Can you work these out from the model? Positions are in its coordinate system, mm. A direction names the side the tool comes from. Round coordinates to 2 decimals unless told otherwise and drop trailing zeros. Loops run counter-clockwise (first coordinate to the right, second up) from the corner with the lowest first, then second, coordinate; pieces in that order, holes last. Notation, with made-up numbers: M -39,-19.5 L -24,-19.5 A21 cw -24,14.5 Z; hole C 14,24.25 d10. An arc over 180 degrees is marked long. Return JSON: item names as keys, results as strings.
```python
from build123d import *

# Parameters (mm, degrees)
CYLINDER003_R           = 1.5
CYLINDER003_DEPTH       = 22
BODY002_PLACEMENT_ANGLE = 180
CYLINDER002_R           = 2
CYLINDER002_DEPTH       = 3


with BuildPart() as cylinder003:
    # Cylinder003 → Cylinder003 (new body)
    with BuildSketch(Plane(origin=(18, 0, 0), x_dir=(0, 0, -1), z_dir=(1, 0, 0))):
        Circle(CYLINDER003_R)
    extrude(amount=CYLINDER003_DEPTH)


with BuildPart() as body002:
    # Sketch002 → Revolution002 (revolve)
    with BuildSketch(Plane.XY):
        Polygon((0, 1.5), (0, 13), (-2, 15), (-8, 15), (-8, 14), (-9, 14), (-9, 12), (-5, 12), (-5, 1.5), align=None)
    revolve(axis=Axis((0, 0, 0), (1, 0, 0)))


with BuildPart() as body002_1:
    # Body002 placement: moved
    add(body002.part.moved(Location((12, 0, 0))).rotate(Axis((12, 0, 0), (0, 0, 1)), BODY002_PLACEMENT_ANGLE))


with BuildPart() as cut:
    # Cylinder002 → Cylinder002 (new body)
    with BuildSketch(Plane(origin=(9, 0, 0), x_dir=(0, 0, -1), z_dir=(1, 0, 0))):
        Circle(CYLINDER002_R)
    extrude(amount=CYLINDER002_DEPTH)

    # Fusion: union Body002
    add(body002_1.part)


with BuildPart() as cut_1:
    # Fusion placement: moved
    add(cut.part.moved(Location((11, 0, 0))))

    # Cut: cut Cylinder003
    add(cylinder003.part, mode=Mode.SUBTRACT)


solid = cut_1.part
```
Q1. Suppose I cut it at B-B, the plane x = 26.25. Please give me the cut outline in (y, z).
Results:
{"outline": "C 0,0 d30; hole C 0,0 d3"}
Q2. I'm going to push flat-ended pins straight in: pin 1 Ø3.5 at (y, z) = (0, 0) entering from +X; pin 2 Ø2 at (x, y) = (28, -5.5) entering from -Z; pin 3 Ø1.5 at (x, z) = (27, 1.5) entering from +Y; pin 4 Ø8 at (y, z) = (9, -4) entering from +X. Where does each tip first touch, or does it pass through?
Results:
{"pin 1": "stops at x = 28", "pin 2": "stops at z = -14.31", "pin 3": "stops at y = 14.98", "pin 4": "stops at x = 32"}
Q3. If I drill on line 1 along Y through (x, z) = (21.4, 0); line 2 along Z through (x, y) = (29.8, 0); line 3 along X through (y, z) = (9, 6), over which ranges is the centre line in solid material (lowest first)?
Results:
{"line 1": "y = -2 to -1.5, 1.5 to 2", "line 2": "z = -15 to -12, 12 to 15", "line 3": "x = 23 to 28"}
Q4. On a 3-axis mill with a long thin cutter (end or side, diameter ignored), from which of +Z, -Z, +X, -X, +Y, -Y can I reach the whole of each face in a straight line? I mean faces 1 (the flat face through (32, 6.3, 10.4)), 2 (the flat face through (28, -2, 0)), 3 (the cylindrical face through (21, -2, 0)). Say none if no direction works.
Results:
{"face 1": "+Z, -Z, +X, +Y, -Y", "face 2": "+X", "face 3": "-X"}
Q5. Suppose I cut it at A-A, the plane x = 24.5. Please give me the cut outline in (y, z), plus the area to 3 significant figures.
Results:
{"outline": "C 0,0 d29; hole C 0,0 d3", "area": "653 mm2"}
Q6. Thinking about a two-plate mould opening in Y: for faces 4 (the cylindrical face through (29.972, 9.523, -7.302)), 5 (the flat face through (23, 3, 0)), 6 (the cylindrical face through (31.51, 3.03, -13.67)), which applies, pulls with the +Y half, pulls with the -Y half, needs draft (parallel to the pull), parting line crosses it, or undercut?
Results:
{"face 4": "undercut", "face 5": "needs draft", "face 6": "parting line crosses it"}
